from build123d import *

# Parameters (mm, degrees)
SKETCH1_R           = 1.5
BOSS_EXTRUDE1_DEPTH = 3


with BuildPart() as part:
    # Sketch1 → Boss-Extrude1 (new body)
    with BuildSketch(Plane(origin=(0, 0, 0), x_dir=(1, 0, 0), z_dir=(0, 1, 0))):
        with BuildLine():
            Line((0, -5), (23.998875872, -5))
            ThreePointArc((23.998875872, -5), (24.467345461, -4.883479623), (24.826642543, -4.561072489))
            Line((24.826642543, -4.561072489), (28.564941326, 0.954149161))
            ThreePointArc((28.564941326, 0.954149161), (28.766036178, 1.172359953), (29.022312673, 1.321950886))
            Line((29.022312673, 1.321950886), (40.929553216, 6.070049343))
            ThreePointArc((40.929553216, 6.070049343), (41.304486381, 6.141164834), (41.678758689, 6.066649533))
            Line((41.678758689, 6.066649533), (47.144586244, 3.829406729))
            Line((47.144586244, 3.829406729), (48.06174016, 3.086958957))
            Line((48.06174016, 3.086958957), (48.804187932, 4.004112872))
            Line((48.804187932, 4.004112872), (49.721341848, 3.2616651))
            Line((49.721341848, 3.2616651), (50.46378962, 4.178819016))
            Line((50.46378962, 4.178819016), (51.380943536, 3.436371244))
            Line((51.380943536, 3.436371244), (52.123391308, 4.35352516))
            Line((52.123391308, 4.35352516), (53.040545224, 3.611077387))
            Line((53.040545224, 3.611077387), (53.782992996, 4.528231303))
            Line((53.782992996, 4.528231303), (54.700146912, 3.785783531))
            Line((54.700146912, 3.785783531), (55.442594685, 4.702937447))
            Line((55.442594685, 4.702937447), (52.341745918, 12.244834503))
            ThreePointArc((52.341745918, 12.244834503), (52.137055639, 12.558350103), (51.831402108, 12.774604725))
            Line((51.831402108, 12.774604725), (46.024183924, 15.419882568))
            ThreePointArc((46.024183924, 15.419882568), (45.628323444, 15.509674561), (45.229386093, 15.434727162))
            Line((45.229386093, 15.434727162), (20.032711481, 5.075121772))
            ThreePointArc((20.032711481, 5.075121772), (19.846254378, 5.018960187), (19.652448068, 5))
            Line((19.652448068, 5), (0, 5))
            ThreePointArc((0, 5), (-5, 0), (0, -5))
        make_face()
        Circle(SKETCH1_R, mode=Mode.SUBTRACT)
        with Locations((22, 0)):
            Circle(SKETCH1_R, mode=Mode.SUBTRACT)
    extrude(amount=BOSS_EXTRUDE1_DEPTH)


solid = part.part
Could you check a few things on this model? Use its own coordinates, in mm. A direction names the side the tool comes from. Give positions to 0.01 mm unless a question says otherwise; leave off trailing zeros. Order: outer loops, then holes, each group sorted by start corner. A loop starts at its lowest first (then second) coordinate and runs counter-clockwise, first axis right, second up. Notation, with made-up numbers: (76, -17) -> (88, -17) arc R19 ccw to (88, 19) -> close; hole circle Ø1 at (79, -18.75). An arc over 180 degrees is marked (long way). Return JSON: item names as keys, results as strings.
1. Imagine slicing it at B-B on x = 22. List the corners of the cut face in (y, z) for me, then the cut area to 3 significant figures.
Answer list:
{"outline": "(0, -5.88) -> (3, -5.88) -> (3, -1.5) -> (0, -1.5) -> close; (0, 1.5) -> (3, 1.5) -> (3, 5) -> (0, 5) -> close", "area": "23.7 mm2"}
2. For pin 1 Ø1.8 at (x, z) = (22, 0) entering from -Y; pin 2 Ø1 at (x, y) = (44.5, 2) entering from +Z; pin 3 Ø1 at (x, y) = (41.5, 2.5) entering from +Z; pin 4 Ø1 at (y, z) = (1.5, 2.5) entering from -X, each with a flat end and sliding along its axis, tell me the tip position at first contact or that it passes through.
Answer list:
{"pin 1": "passes through", "pin 2": "stops at z = -4.71", "pin 3": "stops at z = -5.94", "pin 4": "stops at x = -4.58"}
3. On a 3-axis mill with a long thin cutter (end or side, diameter ignored), from which of +Z, -Z, +X, -X, +Y, -Y can I reach the whole of each face in a straight line? I mean faces 1 (the flat face through (10, 1, -5)), 2 (the flat face through (44.373, 1.479, -4.964)), 3 (the cylindrical face through (20.5, 1.48, -0.07)). Say none if no direction works.
Answer list:
{"face 1": "-Z, -X, +Y, -Y", "face 2": "+Z, +Y, -Y", "face 3": "+Y, -Y"}
4. I need wall thicknesses on line 1 (X direction, y = 0.5, z = 0); line 2 (Z direction, x = 13.5, y = 0.1); line 3 (Z direction, x = -1, y = 2.1). Which ranges of each line are inside material? Lowest first, please. Write a range as from..to.
Answer list:
{"line 1": "x = -5..-1.5, 1.5..20.5, 23.5..27.92", "line 2": "z = -5..5", "line 3": "z = -4.9..-1.12, 1.12..4.9"}
5. Imagine slicing it at A-A on y = 0.7. List the corners of the cut face in (x, z) for me, then the cut area to 3 significant figures.
Answer list:
{"outline": "(0, -5) -> (19.65, -5) arc R1 cw to (20.03, -5.08) -> (45.23, -15.43) arc R1 ccw to (46.02, -15.42) -> (51.83, -12.77) arc R1 ccw to (52.34, -12.24) -> (55.44, -4.7) -> (54.7, -3.79) -> (53.78, -4.53) -> (53.04, -3.61) -> (52.12, -4.35) -> (51.38, -3.44) -> (50.46, -4.18) -> (49.72, -3.26) -> (48.8, -4) -> (48.06, -3.09) -> (47.14, -3.83) -> (41.68, -6.07) arc R1 cw to (40.93, -6.07) -> (29.02, -1.32) arc R1 cw to (28.56, -0.95) -> (24.83, 4.56) arc R1 ccw to (24, 5) -> (0, 5) arc R5 ccw to start; hole circle Ø3 at (0, 0); hole circle Ø3 at (22, 0)", "area": "533 mm2"}
6. Imagine slicing it at C-C on z = 0. List the corners of the cut face in (x, y) for me.
Answer list:
{"outline": "(-5, 0) -> (-1.5, 0) -> (-1.5, 3) -> (-5, 3) -> close; (1.5, 0) -> (20.5, 0) -> (20.5, 3) -> (1.5, 3) -> close; (23.5, 0) -> (27.92, 0) -> (27.92, 3) -> (23.5, 3) -> close"}
7. Imagine slicing it at D-D on x = 32.5. List the corners of the cut face in (y, z) for me.
Answer list:
{"outline": "(0, -10.2) -> (3, -10.2) -> (3, -2.71) -> (0, -2.71) -> close"}
